Here's the drawing with two shaded views (mm, measured from the low corner). I have some questions. A direction names the side the tool comes from. Coordinates: 2 decimals unless noted, no trailing zeros. Loops run counter-clockwise (first coordinate to the right, second up) from the corner with the lowest first, then second, coordinate; pieces in that order, holes last. Notation, with made-up numbers: (-33, 88.25) -> (-4, 88.25) arc R17 cw to (-4, 101.25) -> close; hole circle Ø11 at (16, 44.25). An arc over 180 degrees is marked (long way). Answer as a JSON object with one key per item and string values. Group by question number.
Q1. I want a section at D-D on y = 1.5. Count the separate pieces of the cut face and the enclosed holes in it, then the cut area to 3 significant figures.
Q2. Thinking about a two-plate mould opening in X: for the marked faces 1, 2 and 3, which applies, released by +X, released by -X, zero draft, split by the parting line, or undercut?
Q3. I need wall thicknesses on line 1 (X direction, y = 2.75, z = 11.75) (1 decimal); line 2 (X direction, y = 2.25, z = 8); line 3 (X direction, y = 8, z = 7.75) (1 decimal). Which ranges of each line are inside material? Lowest first, please.
Q4. On a 3-axis mill with a long thin cutter (end or side, diameter ignored), from which of +Z, -Z, +X, -X, +Y, -Y can I reach the whole of each face in a straight line? I mean the marked faces 4 and 5. Say none if no direction works.
Q5. I want a section at B-B on x = 35.5. Write out the boundary of the cut face in (y, z), then the cut area to 3 significant figures.
Q6. I'm going to push flat-ended pins straight in: pin 1 (5.5 mm diameter, centred on x = 34.18, z = 10.05, fed in from -Y); pin 2 (4 mm diameter, centred on x = 11.28, z = 10.05, fed in from -Y). Where does each tip first touch, or does it pass through?
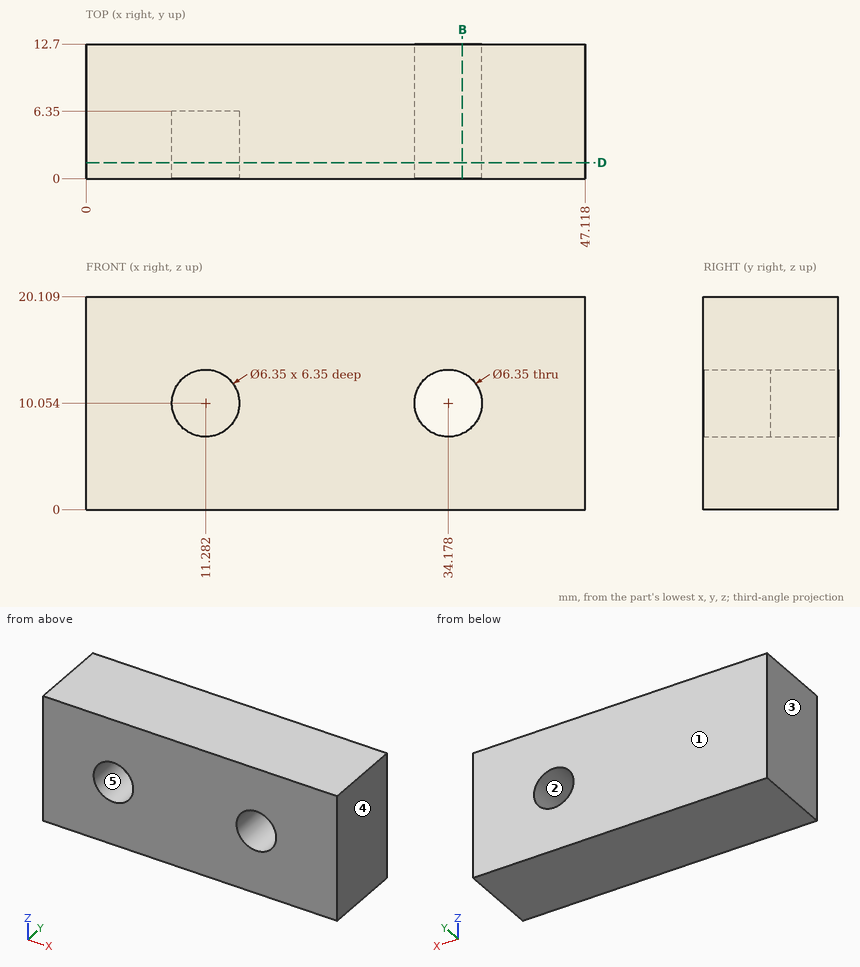
Result set:
{
 "1": {"separate pieces": "1", "enclosed holes": "2", "area": "884 mm²"},
 "2": {"face 1": "zero draft", "face 2": "undercut", "face 3": "released by -X"},
 "3": {"line 1": "x = 0 to 8.6, 14 to 31.5, 36.9 to 47.1", "line 2": "x = 0 to 8.86, 13.7 to 31.76, 36.6 to 47.12", "line 3": "x = 0 to 32, 36.4 to 47.1"},
 "4": {"face 4": "+Z, -Z, +X, +Y, -Y", "face 5": "-Y"},
 "5": {"outline": "(0, 0) -> (12.7, 0) -> (12.7, 7.17) -> (0, 7.17) -> close; (0, 12.94) -> (12.7, 12.94) -> (12.7, 20.11) -> (0, 20.11) -> close", "area": "182 mm²"},
 "6": {"pin 1": "passes through", "pin 2": "stops at y = 6.35"}
}
